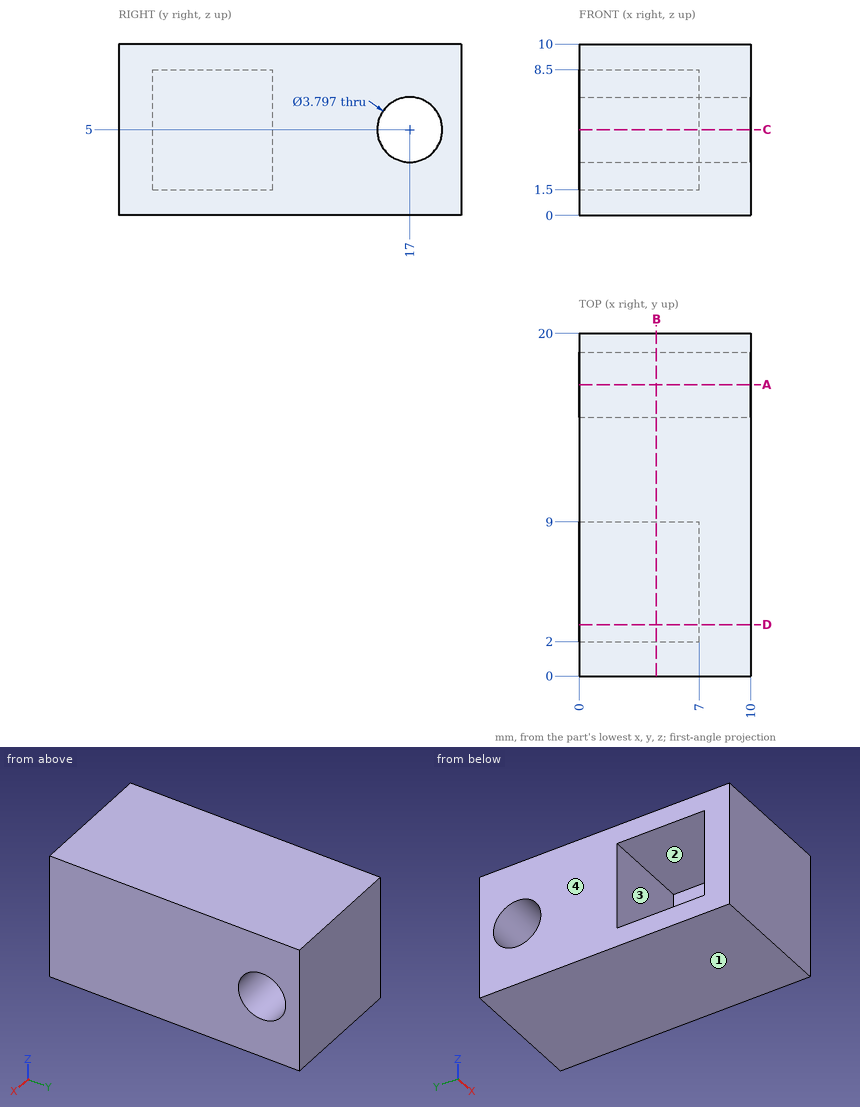
Can you work these out from the drawing? Everything is in mm from the part's minimum corner. Give positions to 0.01 mm unless a question says otherwise; leave off trailing zeros. Order: outer loops, then holes, each group sorted by start corner. A loop starts at its lowest first (then second) coordinate and runs counter-clockwise, first axis right, second up. Notation, with made-up numbers: M -18,28 L 0,28 A19 ccw 0,37 Z; hole C -8.5,5.25 d3. An arc over 180 degrees is marked long. One line per question, with ' | ' between items.
1. I want a section at A-A (y = 17). List the corners of the cut face in (x, z) for me.
Results:
outline: M 0,0 L 10,0 L 10,3.1 L 0,3.1 Z; M 0,6.9 L 10,6.9 L 10,10 L 0,10 Z
2. I want a section at C-C (z = 5). List the corners of the cut face in (x, y) for me.
Results:
outline: M 0,0 L 10,0 L 10,15.1 L 0,15.1 L 0,9 L 7,9 L 7,2 L 0,2 Z; M 0,18.9 L 10,18.9 L 10,20 L 0,20 Z
3. If I drill on line 1 (Y direction, x = 5, z = 5); line 2 (Z direction, x = 6.5, y = 17); line 3 (Z direction, x = 6.75, y = 6), over which ranges is the centre line in solid material (lowest first)?
Results:
line 1: 0 to 2, 9 to 15.1, 18.9 to 20 | line 2: 0 to 3.1, 6.9 to 10 | line 3: 0 to 1.5, 8.5 to 10
4. We'd pull the mould along Z, two halves only. Please class the marked faces 1, 2, 3 and 4: +Z half, -Z half, draft (parallel to the pull), parting line (faces both ways), or undercut.
Results:
face 1: -Z half | face 2: undercut | face 3: undercut | face 4: draft
5. I want a section at B-B (x = 4.5). List the corners of the cut face in (y, z) for me.
Results:
outline: M 0,0 L 20,0 L 20,10 L 0,10 Z; hole M 2,1.5 L 9,1.5 L 9,8.5 L 2,8.5 Z; hole C 17,5 d3.8
6. I'm going to push flat-ended pins straight in: pin 1 (3.5 mm diameter, centred on y = 5.5, z = 5.5, fed in from -X); pin 2 (2.5 mm diameter, centred on y = 17, z = 5, fed in from -X). Where does each tip first touch, or does it pass through?
Results:
pin 1: x = 7 | pin 2: through
7. I want a section at D-D (y = 3). List the corners of the cut face in (x, z) for me, and give its area (3 significant figures).
Results:
outline: M 0,0 L 10,0 L 10,10 L 0,10 L 0,8.5 L 7,8.5 L 7,1.5 L 0,1.5 Z | area: 51.0 mm²
